Could you check a few things on this model? Use its own coordinates, in mm. Face numbers are marked on the shaded views. A direction names the side the tool comes from. Round coordinates to 2 decimals unless told otherwise and drop trailing zeros. Loops run counter-clockwise (first coordinate to the right, second up) from the corner with the lowest first, then second, coordinate; pieces in that order, holes last. Notation, with made-up numbers: M -11.75,36 L 43.25,36 A17 ccw 43.25,65 Z; hole C 4.5,57 d11. An arc over 180 degrees is marked long. Answer in a Markdown table with one row per item.
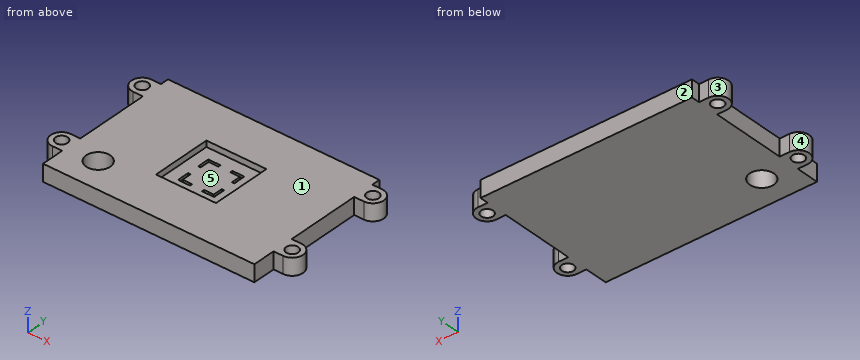
Autodesk Inventor part; units mm, degrees
ref_plane "YZ Plane" through (0, 0, 0) normal (1, 0, 0) x (0, 1, 0)
ref_plane "XZ Plane" through (0, 0, 0) normal (0, 1, 0) x (-1, 0, 0)
ref_plane "XY Plane" through (0, 0, 0) normal (0, 0, 1) x (1, 0, 0)
sketch "Sketch1" plane through (0, 0, 0) normal (0, 0, 1) x (1, 0, 0)
  line L0 (44, -31) -> (-44, -31)
  line L1 (-44, -31) -> (-44, 31)
  line L2 (-44, 31) -> (44, 31)
  line L3 (44, 31) -> (44, -31)
  line L4 (44, -31) -> (-44, 31) construction
  line L5 (-44, -31) -> (44, 31) construction
  point P0 (0, 0)
  dimension "d0" = 88
  dimension "d1" = 62
extrude "Extrusion1" add sketch "Sketch1" along normal blind 7
sketch "Sketch2" plane through (0, 0, 7) normal (0, 0, 1) x (1, 0, 0)
  circle A0 centre (-48, 23) radius 2.5
  line L0 (-48, 23) -> (-44, 23)
  line L1 (-44, 31) -> (-44, -31)
  arc A1 (-48, 27.5) -> (-48, 18.5) centre (-48, 23) ccw
  line L2 (44, 31) -> (-44, 31)
  line L3 (-44, 29.1847) -> (-44, 31)
  line L4 (-44, 16.8153) -> (-44, 18.5)
  line L5 (0, 54.4598) -> (0, -54.4598) construction
  circle A2 centre (48, 23) radius 2.5
  line L6 (48, 23) -> (44, 23)
  line L7 (44, 31) -> (44, -31)
  arc A3 (48, 18.5) -> (48, 27.5) centre (48, 23) ccw
  line L8 (44, 29.1847) -> (44, 31)
  line L9 (44, 16.8153) -> (44, 18.5)
  circle A4 centre (48, -17) radius 2.5
  line L10 (48, -17) -> (44, -17)
  arc A5 (48, -21.5) -> (48, -12.5) centre (48, -17) ccw
  line L11 (44, -10.8153) -> (44, -9)
  line L12 (44, -23.1847) -> (44, -21.5)
  line L13 (-44, 29.1847) -> (-44, 31)
  line L14 (-44, 16.8153) -> (-44, -9)
  line L15 (-44, -23.1847) -> (-44, -31)
  line L16 (44, 29.1847) -> (44, 31)
  line L17 (44, 16.8153) -> (44, -10.8153)
  line L18 (44, -31) -> (44, 31)
  line L19 (44, -23.1847) -> (44, -31)
  line L20 (44, 18.5) -> (48, 18.5)
  line L21 (44, 27.5) -> (48, 27.5)
  line L22 (44, -21.5) -> (48, -21.5)
  line L23 (44, -12.5) -> (48, -12.5)
  line L24 (-48, 27.5) -> (-44, 27.5)
  line L25 (-48, 27.5) -> (-44, 27.5) construction
  line L26 (-48, 18.5) -> (-44, 18.5)
  line L27 (-44, -17) -> (-48, -17)
  circle A6 centre (-48, -17) radius 2.5
  arc A7 (-48, -12.5) -> (-48, -21.5) centre (-48, -17) ccw
  line L28 (-48, -21.5) -> (-44, -21.5)
  line L29 (-48, -12.5) -> (-44, -12.5)
  point P0 (0, 0)
  point P1 (-44, 20.9384)
  point P2 (-44, 25.0616)
  point P3 (-46.6154, 27.2817)
  point P4 (-46.6154, 18.7183)
  point P5 (44, 20.9384)
  point P6 (44, 25.0616)
  point P7 (46.6154, 27.2817)
  point P8 (46.6154, 18.7183)
  point P9 (46.6154, -12.7183)
  point P10 (46.6954, -21.4151)
  point P11 (44, -19.0616)
  point P12 (44, -14.9384)
  point P13 (44, -23.1847)
  dimension "d4" = 5
  dimension "d5" = 4
  dimension "d6" = 2
  dimension "d32" = 8
  dimension "d43" = 4
  dimension "d44" = 5
  dimension "d45" = 2
  dimension "d46" = 40
  dimension "d47" = 0
  dimension "d48" = 5
  dimension "d49" = 2
  dimension "d50" = 40
  dimension "d51" = 4
extrude "Extrusion2" add sketch "Sketch2" against normal blind 7
sketch "Sketch3" plane through (0, 0, 7) normal (0, 0, 1) x (1, 0, 0)
  line L0 (12.5, -12.5) -> (-12.5, -12.5)
  line L1 (-12.5, -12.5) -> (-12.5, 12.5)
  line L2 (-12.5, 12.5) -> (12.5, 12.5)
  line L3 (12.5, 12.5) -> (12.5, -12.5)
  line L4 (12.5, -12.5) -> (-12.5, 12.5) construction
  line L5 (-12.5, -12.5) -> (12.5, 12.5) construction
  point P0 (0, 0)
  dimension "d33" = 25
  dimension "d34" = 25
extrude "Extrusion3" cut sketch "Sketch3" against normal blind 2.5
sketch "Sketch4" plane through (0, 0, 4.5) normal (0, 0, 1) x (1, 0, 0)
  line L0 (-12.5, 12.5) -> (12.5, 12.5)
  line L1 (-12.5, -12.5) -> (-12.5, 12.5)
  line L2 (12.5, -12.5) -> (-12.5, -12.5)
  line L3 (12.5, 12.5) -> (12.5, -12.5)
  line L4 (7.5, 7.5) -> (-7.5, 7.5)
  line L5 (-7.5, 7.5) -> (-7.5, -7.5)
  line L6 (-7.5, -7.5) -> (7.5, -7.5)
  line L7 (7.5, -7.5) -> (7.5, 7.5)
  line L8 (-6.5, 6.5) -> (6.5, 6.5)
  line L9 (6.5, 6.5) -> (6.5, -6.5)
  line L10 (6.5, -6.5) -> (-6.5, -6.5)
  line L11 (-6.5, -6.5) -> (-6.5, 6.5)
  line L12 (-9.9797, 2.5) -> (9.6006, 2.5)
  line L13 (-9.9797, -2.5) -> (9.6006, -2.5)
  line L14 (-2.5, 9.6233) -> (-2.5, -10.0692)
  line L15 (2.5, 9.6233) -> (2.5, -9.2277)
  point P0 (0, 0)
  point P1 (-2.5, -7.5)
  point P2 (-2.5, -6.5)
  point P3 (-6.5, -2.5)
  point P4 (-7.5, -2.5)
  point P5 (2.5, -6.5)
  point P6 (2.5, -7.5)
  point P7 (7.5, -2.5)
  point P8 (6.5, -2.5)
  point P9 (2.5, 7.5)
  point P10 (2.5, 6.5)
  point P11 (6.5, 2.5)
  point P12 (7.5, 2.5)
  point P13 (-2.5, 6.5)
  point P14 (-2.5, 7.5)
  point P15 (-7.5, 2.5)
  point P16 (-6.5, 2.5)
  dimension "d35" = 5
  dimension "d36" = 1
  dimension "d37" = 5
  dimension "d38" = 5
  dimension "d39" = 5
  dimension "d40" = 5
extrude "Extrusion4" cut sketch "Sketch4" against normal blind 1 contours L7 L12 L9 L8 L15 L4 | L14 L8 L11 L12 L5 L4 | L7 L6 L15 L10 L9 L13 | L13 L11 L10 L14 L6 L5
sketch "Sketch5" plane through (0, 0, 0) normal (0, 0, -1) x (-1, 0, 0)
  circle A0 centre (31.5, -18.5) radius 5
  line L0 (44, -21.5) -> (44, -31)
  line L1 (44, -31) -> (-44, -31)
  point P0 (0, 0)
  dimension "d52" = 10
  dimension "d53" = 12.5
  dimension "d54" = 12.5
extrude "Extrusion5" cut sketch "Sketch5" against normal blind 7
properties part number "soporte p2"
1) Will these pins go through, and if not, where does the flat tip stop? P1, Ø1.8, axis at y = 29, z = 2.5, coming from the +X side; P2, Ø3, axis at y = 17.5, z = 2, coming from the +X side; P3, Ø2, axis at x = -46, z = 4, coming from the +Y side.
Computed:
| item | result |
|---|---|
| P1 | stops at x = 44 |
| P2 | stops at x = 50.06 |
| P3 | stops at y = 27.5 |
2) If we mould it in two halves opening along Y, with no side actions, what happens to the marked faces 1, 2 and 3? For each: released by +Y, released by -Y, zero draft, split by the parting line, or undercut.
Computed:
| item | result |
|---|---|
| face 1 | zero draft |
| face 2 | released by +Y |
| face 3 | undercut |
3) Which directions (+Z, -Z, +X, -X, +Y, -Y) give clear straight access to the entire face, cutting with the end or side of a thin tool? Please do the marked faces 4 and 5.
Computed:
| item | result |
|---|---|
| face 4 | +Z, -Z, -X |
| face 5 | +Z |
4) I want a section at B-B, the plane x = -9.5. Please give me the cut outline in (y, z).
Computed:
| item | result |
|---|---|
| outline | M -31,0 L 31,0 L 31,7 L 12.5,7 L 12.5,4.5 L -12.5,4.5 L -12.5,7 L -31,7 Z |
5) I need wall thicknesses on line 1 (Y direction, x = 48, z = 3.25); line 2 (X direction, y = 8, z = 5.75); line 3 (Y direction, x = -31.5, z = 4.5). Which ranges of each line are inside material? Lowest first, please.
Computed:
| item | result |
|---|---|
| line 1 | y = -21.5 to -19.5, -14.5 to -12.5, 18.5 to 20.5, 25.5 to 27.5 |
| line 2 | x = -44 to -12.5, 12.5 to 44 |
| line 3 | y = -31 to -23.5, -13.5 to 31 |
6) I want a section at C-C, the plane y = -18.5. Please give me the cut outline in (x, z), plus the area to 3 significant figures.
Computed:
| item | result |
|---|---|
| outline | M -52.24,0 L -50,0 L -50,7 L -52.24,7 Z; M -46,0 L -36.5,0 L -36.5,7 L -46,7 Z; M -26.5,0 L 46,0 L 46,7 L -26.5,7 Z; M 50,0 L 52.24,0 L 52.24,7 L 50,7 Z |
| area | 605 mm² |
7) I want a section at A-A, the plane z = 1.75. Please give me the cut outline in (x, y), plus the area to 3 significant figures.
Computed:
| item | result |
|---|---|
| outline | M -48,-21.5 L -44,-21.5 L -44,-31 L 44,-31 L 44,-21.5 L 48,-21.5 A4.5 ccw 48,-12.5 L 44,-12.5 L 44,18.5 L 48,18.5 A4.5 ccw 48,27.5 L 44,27.5 L 44,31 L -44,31 L -44,27.5 L -48,27.5 A4.5 ccw -48,18.5 L -44,18.5 L -44,-12.5 L -48,-12.5 A4.5 ccw Z; hole C -48,-17 d5; hole C -48,23 d5; hole C -31.5,-18.5 d10; hole C 48,-17 d5; hole C 48,23 d5 |
| area | 5,570 mm² |
8) I want a section at D-D, the plane y = -8.5. Please give me the cut outline in (x, z).
Computed:
| item | result |
|---|---|
| outline | M -44,0 L 44,0 L 44,7 L 12.5,7 L 12.5,4.5 L -12.5,4.5 L -12.5,7 L -44,7 Z |
